Build history of the part. All positions in model axes, mm. Give positions to 0.01 mm unless a question says otherwise; leave off trailing zeros. Write each loop counter-clockwise with the first axis right and the second up, starting at its lowest first coordinate (ties: lowest second). Pieces come first, ordered by that corner, then holes. Notation, with made-up numbers: (18, 79.25) -> (70, 79.25) arc R11 cw to (70, 89.25) -> close; hole circle Ø9 at (-34.75, 71.25). An arc over 180 degrees is marked (long way). Write item = value, one per line. Start each with the question number.
Q1. Wall check: line 1 (X direction, y = -336.5, z = 9.5); line 2 (X direction, y = -108.5, z = 15); line 3 (X direction, y = -47, z = 4.75). Give the ranges that are in metal, low to high.
Q2. Saw through at A-A, the plane y = -442. List the corners of the cut face in (x, z).
Q3. Drop flat-ended pins along their axis: P1, Ø5.5, axis at y = -318, z = 5.5, coming from the +X side; P2, Ø5.5, axis at x = -6, z = 13, coming from the -Y side; P3, Ø10, axis at y = -347, z = 3, coming from the -X side. Give the stop position or say it passes through.
Q4. Saw through at B-B, the plane z = 13. List the corners of the cut face in (x, y), then the cut area to 3 significant figures.
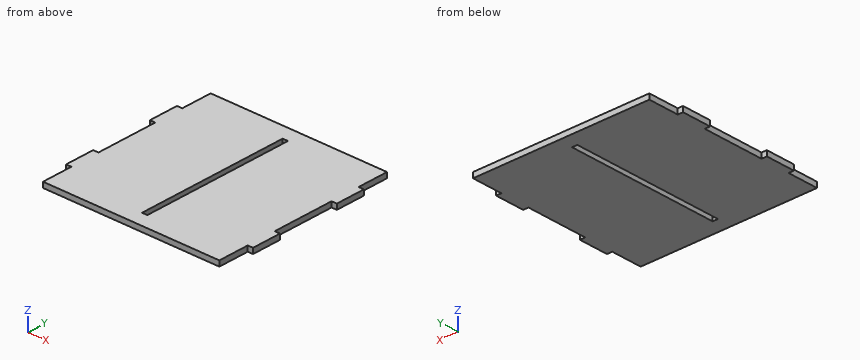
from build123d import *

# Parameters (mm, degrees)
BOSS_EXTRUDE3_DEPTH     = 18
CUT_EXTRUDE1_DEPTH      = 876.584376288
CUT_EXTRUDE1_DEPTH_BACK = 876.584376288
SKETCH2_W               = 18
SKETCH2_H               = 520


with BuildPart() as part:
    # Sketch1 → Boss-Extrude3 (new body)
    with BuildSketch(Plane.XY):
        Polygon((0, 0), (0, -105), (-18, -105), (-18, -205), (0, -205), (0, -415), (-18, -415), (-18, -515), (0, -515), (0, -620), (600, -620), (600, -515), (618, -515), (618, -415), (600, -415), (600, -205), (618, -205), (618, -105), (600, -105), (600, 0), align=None)
    extrude(amount=BOSS_EXTRUDE3_DEPTH)

    # Sketch2 → Cut-Extrude1 (cut, two sides: drawn at the far end of the back side and taken through both)
    with BuildSketch(Plane(origin=(0, 0, 0), x_dir=(-1, 0, 0), z_dir=(0, 0, -1)).offset(-CUT_EXTRUDE1_DEPTH_BACK)):
        with Locations((-300, -310)):
            Rectangle(SKETCH2_W, SKETCH2_H)
    extrude(amount=CUT_EXTRUDE1_DEPTH + CUT_EXTRUDE1_DEPTH_BACK, mode=Mode.SUBTRACT)


solid = part.part
Report:
q1.line_1 = 0 to 291, 309 to 600
q1.line_2 = -18 to 291, 309 to 618
q1.line_3 = 0 to 600
q2.outline = (-18, 0) -> (291, 0) -> (291, 18) -> (-18, 18) -> close; (309, 0) -> (618, 0) -> (618, 18) -> (309, 18) -> close
q3.P1 = 600
q3.P2 = -515
q3.P3 = 0
q4.outline = (-18, -515) -> (0, -515) -> (0, -620) -> (600, -620) -> (600, -515) -> (618, -515) -> (618, -415) -> (600, -415) -> (600, -205) -> (618, -205) -> (618, -105) -> (600, -105) -> (600, 0) -> (0, 0) -> (0, -105) -> (-18, -105) -> (-18, -205) -> (0, -205) -> (0, -415) -> (-18, -415) -> close; hole (291, -570) -> (309, -570) -> (309, -50) -> (291, -50) -> close
q4.area = 370,000 mm2
